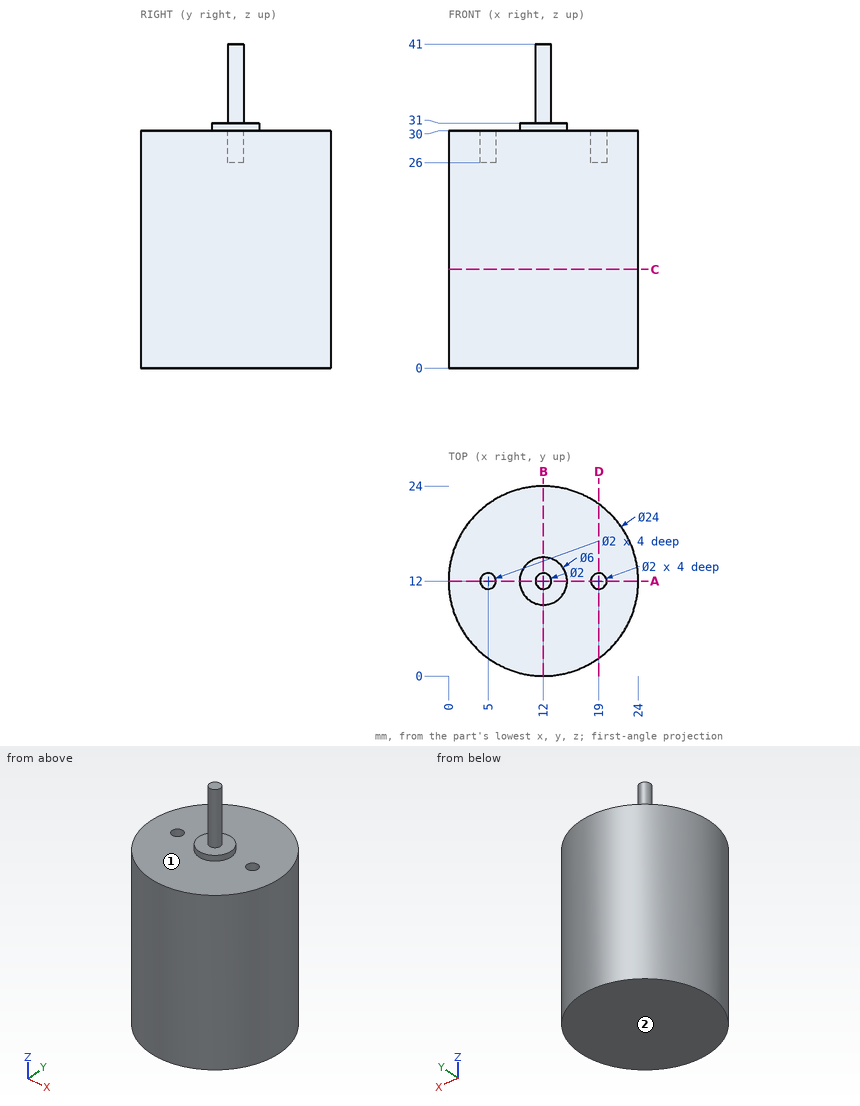
The drawing under review shows one solid part. Ordinate dimensions are in mm from its lowest x, y, z. A direction names the side the tool comes from. Give positions to 0.01 mm unless a question says otherwise; leave off trailing zeros. Order: outer loops, then holes, each group sorted by start corner. A loop starts at its lowest first (then second) coordinate and runs counter-clockwise, first axis right, second up. Notation, with made-up numbers: (-28.5, 75) - (-21.5, 75) arc R14 cw to (-21.5, 92) - close; hole circle Ø3 at (18.25, 47). An arc over 180 degrees is marked (long way). Answer as a JSON object with one key per item and string values. Group by question number.
Item 1: Take a section at D-D on x = 19. Give the boundary of the cut face in (y, z).
Item 2: Machinability: for the marked faces 1 and 2, which of the approach directions +Z, -Z, +X, -X, +Y, -Y give a long, thin tool a straight path to every point of the face, cutting with its end or side? Answer none if there is none.
Item 3: Take a section at A-A on y = 12. Give the boundary of the cut face in (x, z).
Item 4: Clearance check with flat-ended pins moving along their axes: pin 1 Ø5 at (x, z) = (20.5, 5) entering from -Y; pin 2 Ø10 at (x, y) = (17, 17.5) entering from -Z; pin 3 Ø1 at (y, z) = (6, 11) entering from -X; pin 4 Ø4 at (x, z) = (14.5, 6) entering from +Y. State where each tip first meets the part, or that it passes through.
Item 5: Take a section at C-C on z = 12.5. Give the boundary of the cut face in (x, y), and give its area (3 significant figures).
Item 6: Wall thickness on line 1 along Z through (x, y) = (2.75, 7.25); line 2 along Y through (x, z) = (5, 28.35); line 3 along Y through (x, z) = (12.5, 10): over which ranges is each line inside the solid? List them lowest first.
Item 7: Take a section at B-B on x = 12. Give the boundary of the cut face in (y, z).
Reported:
{
 "1": {"outline": "(2.25, 0) - (21.75, 0) - (21.75, 30) - (13, 30) - (13, 26) - (11, 26) - (11, 30) - (2.25, 30) - close"},
 "2": {"face 1": "+Z", "face 2": "-Z, +X, -X, +Y, -Y"},
 "3": {"outline": "(0, 0) - (24, 0) - (24, 30) - (20, 30) - (20, 26) - (18, 26) - (18, 30) - (15, 30) - (15, 31) - (13, 31) - (13, 41) - (11, 41) - (11, 31) - (9, 31) - (9, 30) - (6, 30) - (6, 26) - (4, 26) - (4, 30) - (0, 30) - close"},
 "4": {"pin 1": "y = 1.61", "pin 2": "z = 0", "pin 3": "x = 1.33", "pin 4": "y = 23.99"},
 "5": {"outline": "circle Ø24 at (12, 12)", "area": "452 mm^2"},
 "6": {"line 1": "0 to 30", "line 2": "2.25 to 11, 13 to 21.75", "line 3": "0.01 to 23.99"},
 "7": {"outline": "(0, 0) - (24, 0) - (24, 30) - (15, 30) - (15, 31) - (13, 31) - (13, 41) - (11, 41) - (11, 31) - (9, 31) - (9, 30) - (0, 30) - close"}
}
